Model file for the job. Use its own axes, mm. Face numbers are marked on the shaded views. A direction names the side the tool comes from. Coordinates: 2 decimals unless noted, no trailing zeros. Order: outer loops, then holes, each group sorted by start corner. A loop starts at its lowest first (then second) coordinate and runs counter-clockwise, first axis right, second up. Notation, with made-up numbers: (71.5, 69.25) -> (117.5, 69.25) arc R21 cw to (117.5, 73.25) -> close; hole circle Ø2 at (59, -15). An arc over 180 degrees is marked (long way). Use CSV: the item, a comma, the result in double quotes. Start each with the question number.
(1) Cut at A-A on x = 0. Write the cut outline in (y, z).
(2) Cut at B-B on z = 0. Write the cut outline in (x, y), plus the area to 3 significant figures.
(3) Tool access for the marked faces 1 and 2: list every direction of +Z, -Z, +X, -X, +Y, -Y with a clear straight run to the whole face (end or side of a thin tool).
(4) Cut at C-C on y = -4.25. Write the cut outline in (x, z), plus the area to 3 significant figures.
(5) Pin check, flat tips, straight feed: pin 1 Ø1 at (x, y) = (-3.5, 0) entering from +Z; pin 2 Ø11 at (x, z) = (3, -3.5) entering from +Y; pin 3 Ø2 at (y, z) = (1, -2) entering from -X; pin 4 Ø1.5 at (x, y) = (4.5, 0) entering from -Z. Stop position of each tip, or through.
(6) Probe L1, parallel to Y at x = 9.25, z = -1.25; L2, parallel to X at y = -1.25, z = 1; L3, parallel to X at y = 2, z = 0. List the from-to ranges inside material, lowest first.
(7) Cut at D-D on y = -3. Write the cut outline in (x, z).
```python
from build123d import *

# Parameters (mm, degrees)
SKETCH1_R           = 4.05
BOSS_EXTRUDE1_DEPTH = 3.5
FILLET1_R           = 0.79375
SKETCH2_R           = 11
BOSS_EXTRUDE2_DEPTH = 2


with BuildPart() as part:
    # Sketch1 → Boss-Extrude1 (new body, symmetric)
    with BuildSketch(Plane(origin=(0, 0, 0), x_dir=(1, 0, 0), z_dir=(0, 1, 0))):
        Circle(SKETCH1_R)
    extrude(amount=BOSS_EXTRUDE1_DEPTH, both=True)

    # Fillet1
    fillet1_edges = [part.edges().sort_by_distance(p)[0] for p in [
        (-4.05, 3.5, 0),
    ]]
    fillet(fillet1_edges, radius=FILLET1_R)

    # Sketch2 → Boss-Extrude2 (add)
    with BuildSketch(Plane.XZ.offset(3.5)):
        Circle(SKETCH2_R)
    extrude(amount=BOSS_EXTRUDE2_DEPTH)


solid = part.part
```
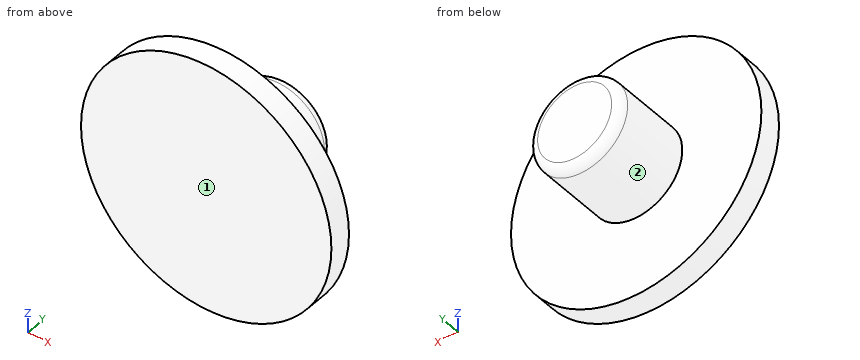
Outcome:
1,outline,"(-5.5, -11) -> (-3.5, -11) -> (-3.5, -4.05) -> (2.71, -4.05) arc R0.79 ccw to (3.5, -3.26) -> (3.5, 3.26) arc R0.79 ccw to (2.71, 4.05) -> (-3.5, 4.05) -> (-3.5, 11) -> (-5.5, 11) -> close"
2,outline,"(-11, -5.5) -> (11, -5.5) -> (11, -3.5) -> (4.05, -3.5) -> (4.05, 2.71) arc R0.79 ccw to (3.26, 3.5) -> (-3.26, 3.5) arc R0.79 ccw to (-4.05, 2.71) -> (-4.05, -3.5) -> (-11, -3.5) -> close"
2,area,"100 mm2"
3,face 1,"+Z, -Z, +X, -X, -Y"
3,face 2,"+Y"
4,outline,"circle Ø22 at (0, 0)"
4,area,"380 mm2"
5,pin 1,"z = 2.72"
5,pin 2,"y = 3.5"
5,pin 3,"x = -3.92"
5,pin 4,"z = -1.53"
6,L1,"-5.5 to -3.5"
6,L2,"-3.92 to 3.92"
6,L3,"-4.05 to 4.05"
7,outline,"circle Ø8.1 at (0, 0)"
